```python
from build123d import *

# Parameters (mm, degrees)
SKETCH2_R          = 3.25
CUT_EXTRUDE1_DEPTH = 74.98310618
CIRPATTERN1_COUNT  = 6


with BuildPart() as part:
    # Sketch1 → Revolve1 (revolve)
    with BuildSketch(Plane(origin=(0, 0, 0), x_dir=(0, 0, -1), z_dir=(1, 0, 0)), mode=Mode.PRIVATE) as revolve1_sk:
        Polygon((-31, 47.5), (0, 47.5), (0, 26), (-19, 26), (-19, 20), (-31, 20), align=None)
    revolve(revolve1_sk.sketch.rotate(Axis((0, 0, 0), (0, 0, 1)), 90), axis=Axis((0, 0, 0), (0, 0, 1)))

    # Sketch2 → Cut-Extrude1 (cut, through all)
    with BuildSketch(Plane.XY.offset(31)):
        with Locations((0, 37.25)):
            Circle(SKETCH2_R)
    cut_extrude1 = extrude(amount=-CUT_EXTRUDE1_DEPTH, mode=Mode.SUBTRACT)

    # CirPattern1: Cut-Extrude1 ×6 about axis
    cirpattern1_axis = Axis((0, 0, 0), (0, 0, 1))
    for i in range(1, CIRPATTERN1_COUNT):
        add(cut_extrude1.rotate(cirpattern1_axis, i * 360 / CIRPATTERN1_COUNT), mode=Mode.SUBTRACT)


solid = part.part
```
Work out the finished part from the listing and answer in its coordinate system (mm). A direction names the side the tool comes from. Round coordinates to 2 decimals unless told otherwise and drop trailing zeros. Write each loop counter-clockwise with the first axis right and the second up, starting at its lowest first coordinate (ties: lowest second). Pieces come first, ordered by that corner, then holes. Notation, with made-up numbers: (36, -6.5) - (57, -6.5) arc R18 ccw to (57, 2.5) - close; hole circle Ø6 at (49.25, 29.25). An arc over 180 degrees is marked (long way). Return JSON: item names as keys, results as strings. Group by question number.
Q1. Each of these flat-tipped pins is pushed along its axis until it touches: pin 1 Ø5 at (y, z) = (-30.5, 15.5) entering from +X; pin 2 Ø4 at (y, z) = (6, 25) entering from -X; pin 3 Ø8 at (x, y) = (-13.5, -9) entering from -Z. Where does it stop, or does it pass through?
Q2. The part is cut by section A-A on y = 0. Write down the section's boundary in (x, z).
Q3. The mould has two halves that part along X. Classify faces 1 (the flat face through (20.4, -0.7, 31)), 2 (the cylindrical face through (10.3, 46.37, 15.28)), 3 (the cylindrical face through (-31.555, 21.798, 15.717)): released by +X, released by -X, zero draft, split by the parting line, or undercut.
Q4. Find the intervals of material crossed by L1, parallel to Y at x = 0, z = 13; L2, parallel to Y at x = 0, z = 20; L3, parallel to Y at x = -31.5, z = 19, in increasing order.
Q5. For faces 4 (the cylindrical face through (0.705, -34.077, 15.717)), 5 (the cylindrical face through (20.633, 15.821, 9.633)), determine the directions among +Z, -Z, +X, -X, +Y, -Y from which every point of the face is accessible in a straight line to the end or side of a thin tool.
Q6. The part is cut by section C-C on y = 23.5. Write down the section's boundary in (x, z).
Q7. The part is cut by section B-B on x = 0. Write down the section's boundary in (y, z), then the cut area to 3 significant figures.
Solved:
{
 "1": {"pin 1": "x = 38.37", "pin 2": "x = -47.33", "pin 3": "z = 19"},
 "2": {"outline": "(-47.5, 0) - (-26, 0) - (-26, 19) - (-20, 19) - (-20, 31) - (-47.5, 31) - close; (20, 19) - (26, 19) - (26, 0) - (47.5, 0) - (47.5, 31) - (20, 31) - close"},
 "3": {"face 1": "zero draft", "face 2": "split by the parting line", "face 3": "undercut"},
 "4": {"L1": "-47.5 to -40.5, -34 to -26, 26 to 34, 40.5 to 47.5", "L2": "-47.5 to -40.5, -34 to -20, 20 to 34, 40.5 to 47.5", "L3": "-35.55 to -21.79, -15.46 to 15.46, 21.79 to 35.55"},
 "5": {"face 4": "+Z, -Z", "face 5": "-Z"},
 "6": {"outline": "(-41.28, 0) - (-11.12, 0) - (-11.12, 19) - (11.12, 19) - (11.12, 0) - (41.28, 0) - (41.28, 31) - (-41.28, 31) - close"},
 "7": {"outline": "(-47.5, 0) - (-40.5, 0) - (-40.5, 31) - (-47.5, 31) - close; (-34, 0) - (-26, 0) - (-26, 19) - (-20, 19) - (-20, 31) - (-34, 31) - close; (20, 19) - (26, 19) - (26, 0) - (34, 0) - (34, 31) - (20, 31) - close; (40.5, 0) - (47.5, 0) - (47.5, 31) - (40.5, 31) - close", "area": "1,070 mm²"}
}
